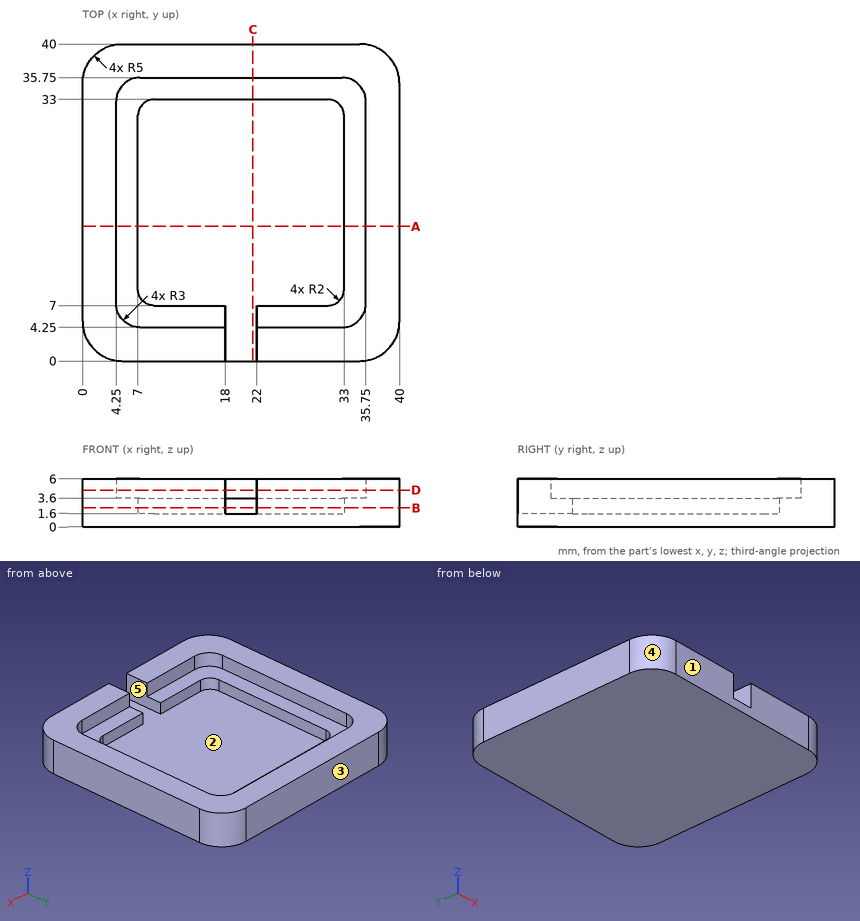
The figure shows three views and two pictorial views of one solid part (mm, origin at its lowest corner). Answer the questions. A direction names the side the tool comes from. Give positions to 0.01 mm unless a question says otherwise; leave off trailing zeros. Write each loop counter-clockwise with the first axis right and the second up, starting at its lowest first coordinate (ties: lowest second). Pieces come first, ordered by that corner, then holes. Notation, with made-up numbers: (39.25, -4) - (48.25, -4) arc R34 ccw to (48.25, 28) - close; hole circle Ø9 at (76, -34). An arc over 180 degrees is marked (long way). Use CSV: the item, a comma, the result in double quotes. Start each with the question number.
Item 1: The part is cut by section B-B, the plane z = 2.35. Give the vertices of the cut face in (x, y), and give its area (3 significant figures).
Item 2: The part is cut by section C-C, the plane x = 21.5. Give the vertices of the cut face in (y, z).
Item 3: The mould has two halves that part along Y. Classify the marked faces 1, 2 and 3: pulls with the +Y half, pulls with the -Y half, needs draft (parallel to the pull), parting line crosses it, or undercut.
Item 4: The part is cut by section D-D, the plane z = 4.6. Give the vertices of the cut face in (x, y), and give its area (3 significant figures).
Item 5: Flat-ended cylindrical pins translate along their axes: P1, Ø3.5, axis at y = 2, z = 3.5, coming from the +X side; P2, Ø3.5, axis at y = 3, z = 4.5, coming from the -X side; P3, Ø8, axis at x = 23, y = 21, coming from the +Z side. Find the tip coordinate at first contact, or state that the pin passes through.
Item 6: Consider line 1 (X direction, y = 23.5, z = 2.45); line 2 (X direction, y = 30.5, z = 5.25). Determine where each line is inside the solid, lowest interval first.
Item 7: The part is cut by section A-A, the plane y = 17. Give the vertices of the cut face in (x, z).
Item 8: For the marked faces 4 and 5, determine the directions among +Z, -Z, +X, -X, +Y, -Y from which every point of the face is accessible in a straight line to the end or side of a thin tool.
Taken from the geometry:
1,outline,"(0, 5) arc R5 ccw to (5, 0) - (18, 0) - (18, 7) - (9, 7) arc R2 cw to (7, 9) - (7, 31) arc R2 cw to (9, 33) - (31, 33) arc R2 cw to (33, 31) - (33, 9) arc R2 cw to (31, 7) - (22, 7) - (22, 0) - (35, 0) arc R5 ccw to (40, 5) - (40, 35) arc R5 ccw to (35, 40) - (5, 40) arc R5 ccw to (0, 35) - close"
1,area,"878 mm2"
2,outline,"(0, 0) - (40, 0) - (40, 6) - (35.75, 6) - (35.75, 3.6) - (33, 3.6) - (33, 1.6) - (0, 1.6) - close"
3,face 1,"pulls with the -Y half"
3,face 2,"undercut"
3,face 3,"pulls with the +Y half"
4,outline,"(0, 5) arc R5 ccw to (5, 0) - (18, 0) - (18, 4.25) - (7.25, 4.25) arc R3 cw to (4.25, 7.25) - (4.25, 32.75) arc R3 cw to (7.25, 35.75) - (32.75, 35.75) arc R3 cw to (35.75, 32.75) - (35.75, 7.25) arc R3 cw to (32.75, 4.25) - (22, 4.25) - (22, 0) - (35, 0) arc R5 ccw to (40, 5) - (40, 35) arc R5 ccw to (35, 40) - (5, 40) arc R5 ccw to (0, 35) - close"
4,area,"577 mm2"
5,P1,"x = 39.84"
5,P2,"x = 0.01"
5,P3,"z = 1.6"
6,line 1,"0 to 7, 33 to 40"
6,line 2,"0 to 4.25, 35.75 to 40"
7,outline,"(0, 0) - (40, 0) - (40, 6) - (35.75, 6) - (35.75, 3.6) - (33, 3.6) - (33, 1.6) - (7, 1.6) - (7, 3.6) - (4.25, 3.6) - (4.25, 6) - (0, 6) - close"
8,face 4,"+Z, -Z, -X, -Y"
8,face 5,"+Z, -Y"
